```python
from build123d import *

# Parameters (mm, degrees)
F1_DEPTH = 30
F2_DEPTH = 10
F3_SIZE  = 0.5


with BuildPart() as f1:
    # F0 (on Front) → F1 (new body)
    with BuildSketch(Plane.XZ):
        with BuildLine():
            Line((-0.25, 2.8892040426), (-0.25, 3.9921798557))
            ThreePointArc((-0.25, 3.9921798557), (-4, 0), (-0.25, -3.9921798557))
            Line((-0.25, -3.9921798557), (-0.25, -2.8892040426))
            ThreePointArc((-0.25, -2.8892040426), (-2.9, 0), (-0.25, 2.8892040426))
        make_face()
    extrude(amount=-F1_DEPTH)



with BuildPart() as f1b:
    # F0 (on Front) → F1, piece 2 (new body)
    with BuildSketch(Plane.XZ):
        with BuildLine():
            ThreePointArc((0.25, -3.9921798557), (2.9154759474, -2.7386127875), (4, 0))
            ThreePointArc((4, 0), (2.9154759474, 2.7386127875), (0.25, 3.9921798557))
            Line((0.25, 3.9921798557), (0.25, 2.8892040426))
            ThreePointArc((0.25, 2.8892040426), (2.1371710273, 1.9602295784), (2.9, 0))
            ThreePointArc((2.9, 0), (2.1371710273, -1.9602295784), (0.25, -2.8892040426))
            Line((0.25, -2.8892040426), (0.25, -3.9921798557))
        make_face()
    extrude(amount=-F1_DEPTH)


with BuildPart() as f1_1:
    add(f1.part)

    add(f1b.part)  # F2 merges F1b
    # F0 (on Front) → F2 (join)
    with BuildSketch(Plane.XZ):
        with BuildLine():
            ThreePointArc((0.25, -3.9921798557), (2.9154759474, -2.7386127875), (4, 0))
            ThreePointArc((4, 0), (2.9154759474, 2.7386127875), (0.25, 3.9921798557))
            Line((0.25, 3.9921798557), (0.25, 2.8892040426))
            ThreePointArc((0.25, 2.8892040426), (2.1371710273, 1.9602295784), (2.9, 0))
            ThreePointArc((2.9, 0), (2.1371710273, -1.9602295784), (0.25, -2.8892040426))
            Line((0.25, -2.8892040426), (0.25, -3.9921798557))
        make_face()
        with BuildLine():
            Line((0.25, 2.8892040426), (0.25, 3.9921798557))
            ThreePointArc((0.25, 3.9921798557), (0, 4), (-0.25, 3.9921798557))
            Line((-0.25, 3.9921798557), (-0.25, 2.8892040426))
            ThreePointArc((-0.25, 2.8892040426), (0, 2.9), (0.25, 2.8892040426))
        make_face()
        with BuildLine():
            ThreePointArc((-0.25, -3.9921798557), (0, -4), (0.25, -3.9921798557))
            Line((0.25, -3.9921798557), (0.25, -2.8892040426))
            ThreePointArc((0.25, -2.8892040426), (0, -2.9), (-0.25, -2.8892040426))
            Line((-0.25, -2.8892040426), (-0.25, -3.9921798557))
        make_face()
        with BuildLine():
            Line((-0.25, 2.8892040426), (-0.25, 3.9921798557))
            ThreePointArc((-0.25, 3.9921798557), (-4, 0), (-0.25, -3.9921798557))
            Line((-0.25, -3.9921798557), (-0.25, -2.8892040426))
            ThreePointArc((-0.25, -2.8892040426), (-2.9, 0), (-0.25, 2.8892040426))
        make_face()
    extrude(amount=F2_DEPTH)

    # F3
    f3_edges = [f1_1.edges().sort_by_distance(p)[0] for p in [
        (-2.9, 30, 0),
        (2.9, 30, 0),
    ]]
    chamfer(f3_edges, length=F3_SIZE)


solid = f1_1.part
```
Read the model definition and answer for the solid it produces. Units are mm, in the model's axes. A direction names the side the tool comes from. Round coordinates to 2 decimals unless told otherwise and drop trailing zeros. One line per item, written item: value.
Q1. Flat-ended cylindrical pins translate along their axes: pin 1 Ø1 at (y, z) = (16, 2) entering from +X; pin 2 Ø1.5 at (x, y) = (-2.5, 24) entering from +Z; pin 3 Ø1.2 at (y, z) = (14, -3) entering from +X. Find the tip coordinate at first contact, or state that the pin passes through.
Data:
pin 1: x = 3.71
pin 2: z = 3.6
pin 3: x = 3.2
Q2. For a pull along X with two mould halves and no side action, classify faces 1 (the flat face through (3.5, 30, -0.6)), 2 (the cylindrical face through (0.425, 10.28, 3.977)), 3 (the conical face through (-3.04, 29.64, -0.06)) as +X half, -X half, draft (parallel to the pull), parting line (faces both ways), or undercut.
Data:
face 1: draft
face 2: parting line
face 3: undercut
Q3. Straight lines are drawn through the part: line 1 (X direction, y = -3.5, z = 0.25); line 2 (Z direction, x = -1, y = -1); line 3 (Z direction, x = 1.75, y = -5). For each, find the intervals that lie inside material, in ascending order. Write a range as [from, to].
Data:
line 1: [-3.99, -2.89], [2.89, 3.99]
line 2: [-3.87, -2.72], [2.72, 3.87]
line 3: [-3.6, -2.31], [2.31, 3.6]
Q4. Which of the six approach directions +Z, -Z, +X, -X, +Y, -Y give full straight-line access (tool end or side, diameter ignored) to faces 4 (the flat face through (-3.5, 30, -0.6)), 5 (the flat face through (-0.25, 14.8, 3.4))?
Data:
face 4: +Z, -Z, +X, -X, +Y
face 5: +Z, -Z, +Y
